Source: CAD feature listing. Evaluate the final solid. Frame: model axes, mm. A direction names the side the tool comes from. Coordinates: 2 decimals unless noted, no trailing zeros. Order: outer loops, then holes, each group sorted by start corner. A loop starts at its lowest first (then second) coordinate and runs counter-clockwise, first axis right, second up. Notation, with made-up numbers: (41.25, 26.25) -> (97.25, 26.25) arc R22 ccw to (97.25, 57.25) -> close; hole circle Ø2 at (53, 75). An arc over 180 degrees is marked (long way). Put each result on its own line as item: value.
from build123d import *

# Parameters (mm, degrees)
SKETCH_W        = 50
SKETCH_H        = 55
PAD_DEPTH       = 4
PAD001_DEPTH    = 50
SKETCH002_R     = 11
POCKET_DEPTH    = 5
SKETCH003_R     = 1.6
POCKET001_DEPTH = 50
SKETCH004_W     = 54
SKETCH004_H     = 63
PAD002_DEPTH    = 4
SKETCH005_R     = 2.1
POCKET002_DEPTH = 60
POCKET003_DEPTH = 5
POCKET004_DEPTH = 70
SKETCH008_W     = 45
SKETCH008_H     = 45
POCKET005_DEPTH = 5


with BuildPart() as part:
    # Sketch → Pad (new body)
    with BuildSketch(Plane.XY):
        with Locations((25, 27.5)):
            Rectangle(SKETCH_W, SKETCH_H)
    extrude(amount=PAD_DEPTH)

    # Sketch001 (on Face6 of Pad) → Pad001 (join)
    with BuildSketch(Plane.XY.offset(4)):
        Polygon((50, 55), (50, 59), (-4, 59), (-4, -4), (50, -4), (50, 0), (0, 0), (0, 55), align=None)
    extrude(amount=-PAD001_DEPTH)

    # Sketch002 (on Face4 of Pad001) → Pocket (cut)
    with BuildSketch(Plane(origin=(0, 0, 0), x_dir=(1, 0, 0), z_dir=(0, 0, -1))):
        with Locations((25, -25)):
            Circle(SKETCH002_R)
    extrude(amount=-POCKET_DEPTH, mode=Mode.SUBTRACT)

    # Sketch003 (on Face5 of Pocket) → Pocket001 (cut)
    with BuildSketch(Plane.XY.offset(4)):
        with Locations((40.5, 40.5)):
            Circle(SKETCH003_R)
        with Locations((40.5, 9.5)):
            Circle(SKETCH003_R)
        with Locations((9.5, 9.5)):
            Circle(SKETCH003_R)
        with Locations((9.5, 40.5)):
            Circle(SKETCH003_R)
    extrude(amount=-POCKET001_DEPTH, mode=Mode.SUBTRACT)

    # Sketch004 (on DatumPlane) → Pad002 (join)
    with BuildSketch(Plane(origin=(0, 0, -46), x_dir=(1, 0, 0), z_dir=(0, 0, -1))):
        with Locations((23, -27.5)):
            Rectangle(SKETCH004_W, SKETCH004_H)
    extrude(amount=PAD002_DEPTH)

    # Sketch005 (on Face22 of Pad002) → Pocket002 (cut)
    with BuildSketch(Plane(origin=(0, 0, -50), x_dir=(1, 0, 0), z_dir=(0, 0, -1))):
        with Locations((5, -5)):
            Circle(SKETCH005_R)
        with Locations((45, -5)):
            Circle(SKETCH005_R)
        with Locations((45, -51)):
            Circle(SKETCH005_R)
        with Locations((5, -51)):
            Circle(SKETCH005_R)
    extrude(amount=-POCKET002_DEPTH, mode=Mode.SUBTRACT)

    # Sketch006 (on Face22 of Pocket002) → Pocket003 (cut)
    with BuildSketch(Plane(origin=(-4, 0, 0), x_dir=(0, -1, 0), z_dir=(-1, 0, 0))):
        with BuildLine():
            ThreePointArc((-48, -10), (-49.5, -11.5), (-48, -13))
            Line((-48, -13), (-8, -13))
            ThreePointArc((-8, -13), (-6.5, -11.5), (-8, -10))
            Line((-8, -10), (-48, -10))
        make_face()
        with BuildLine():
            ThreePointArc((-48, -24.994244), (-49.5, -26.494244), (-48, -27.994244))
            Line((-48, -27.994244), (-8, -27.994244))
            ThreePointArc((-8, -27.994244), (-6.5, -26.494244), (-8, -24.994244))
            Line((-8, -24.994244), (-48, -24.994244))
        make_face()
        with BuildLine():
            ThreePointArc((-47.876909, -14.998485), (-49.376909, -16.498485), (-47.876909, -17.998485))
            Line((-47.876909, -17.998485), (-7.876909, -17.998485))
            ThreePointArc((-7.876909, -17.998485), (-6.376909, -16.498485), (-7.876909, -14.998485))
            Line((-7.876909, -14.998485), (-47.876909, -14.998485))
        make_face()
        with BuildLine():
            ThreePointArc((-48.0704, -19.994739), (-49.5704, -21.494739), (-48.0704, -22.994739))
            Line((-48.0704, -22.994739), (-8.0704, -22.994739))
            ThreePointArc((-8.0704, -22.994739), (-6.5704, -21.494739), (-8.0704, -19.994739))
            Line((-8.0704, -19.994739), (-48.0704, -19.994739))
        make_face()
        with BuildLine():
            ThreePointArc((-48, -34.994244), (-49.5, -36.494244), (-48, -37.994244))
            Line((-48, -37.994244), (-8, -37.994244))
            ThreePointArc((-8, -37.994244), (-6.5, -36.494244), (-8, -34.994244))
            Line((-8, -34.994244), (-48, -34.994244))
        make_face()
        with BuildLine():
            ThreePointArc((-48, -29.994244), (-49.5, -31.494244), (-48, -32.994244))
            Line((-48, -32.994244), (-8, -32.994244))
            ThreePointArc((-8, -32.994244), (-6.5, -31.494244), (-8, -29.994244))
            Line((-8, -29.994244), (-48, -29.994244))
        make_face()
    extrude(amount=-POCKET003_DEPTH, mode=Mode.SUBTRACT)

    # Sketch007 (on Face11 of Pocket003) → Pocket004 (cut)
    with BuildSketch(Plane(origin=(0, 59, 0), x_dir=(-1, 0, 0), z_dir=(0, 1, 0))):
        with BuildLine():
            ThreePointArc((-35, -8.5), (-36.5, -10), (-35, -11.5))
            Line((-35, -11.5), (-10, -11.5))
            ThreePointArc((-10, -11.5), (-8.5, -10), (-10, -8.5))
            Line((-10, -8.5), (-35, -8.5))
        make_face()
        with BuildLine():
            ThreePointArc((-35, -14.5), (-36.5, -16), (-35, -17.5))
            Line((-35, -17.5), (-10, -17.5))
            ThreePointArc((-10, -17.5), (-8.5, -16), (-10, -14.5))
            Line((-10, -14.5), (-35, -14.5))
        make_face()
        with BuildLine():
            ThreePointArc((-35, -20.53228), (-36.5, -22.03228), (-35, -23.53228))
            Line((-35, -23.53228), (-10, -23.53228))
            ThreePointArc((-10, -23.53228), (-8.5, -22.03228), (-10, -20.53228))
            Line((-10, -20.53228), (-35, -20.53228))
        make_face()
        with BuildLine():
            ThreePointArc((-35, -26.484331), (-36.5, -27.984331), (-35, -29.484331))
            Line((-35, -29.484331), (-10, -29.484331))
            ThreePointArc((-10, -29.484331), (-8.5, -27.984331), (-10, -26.484331))
            Line((-10, -26.484331), (-35, -26.484331))
        make_face()
        with BuildLine():
            ThreePointArc((-35, -32.449028), (-36.5, -33.949028), (-35, -35.449028))
            Line((-35, -35.449028), (-10, -35.449028))
            ThreePointArc((-10, -35.449028), (-8.5, -33.949028), (-10, -32.449028))
            Line((-10, -32.449028), (-35, -32.449028))
        make_face()
        with BuildLine():
            ThreePointArc((-35, -38.428181), (-36.5, -39.928181), (-35, -41.428181))
            Line((-35, -41.428181), (-10, -41.428181))
            ThreePointArc((-10, -41.428181), (-8.5, -39.928181), (-10, -38.428181))
            Line((-10, -38.428181), (-35, -38.428181))
        make_face()
    extrude(amount=-POCKET004_DEPTH, mode=Mode.SUBTRACT)

    # Sketch008 (on Face50 of Pocket004) → Pocket005 (cut)
    with BuildSketch(Plane(origin=(0, 0, -50), x_dir=(1, 0, 0), z_dir=(0, 0, -1))):
        with Locations((25, -25)):
            Rectangle(SKETCH008_W, SKETCH008_H)
    extrude(amount=-POCKET005_DEPTH, mode=Mode.SUBTRACT)


solid = part.part
1. First-contact query: pin 1 (3 mm diameter, centred on y = 52.5, z = -13, fed in from +X); pin 2 (15 mm diameter, centred on x = 31, y = 30.5, fed in from -Z). Flat tips, straight axial feed; report the tip coordinate or a pass-through.
Numbers:
pin 1: stops at x = 0
pin 2: stops at z = 0
2. Cut plane A-A on x = 40.5. Output: boundary loops of the cut face in (y, z).
Numbers:
outline: (-4, -50) -> (2.5, -50) -> (2.5, -46) -> (0, -46) -> (0, 0) -> (7.9, 0) -> (7.9, 4) -> (-4, 4) -> close; (11.1, 0) -> (38.9, 0) -> (38.9, 4) -> (11.1, 4) -> close; (42.1, 0) -> (55, 0) -> (55, -46) -> (47.5, -46) -> (47.5, -50) -> (59, -50) -> (59, 4) -> (42.1, 4) -> close
3. Set-up query: faces 4 (the flat face through (-2, 28, -10)), 5 (the cylindrical face through (8.5, -2, -40)), 6 (the cylindrical face through (45.969, 52.863, -48.028)). Return all of +Z, -Z, +X, -X, +Y, -Y with unobstructed straight access to the full face (end or side cutting, diameter ignored); none if empty.
Numbers:
face 4: +X, -X
face 5: +Y, -Y
face 6: +Z, -Z
4. Cut plane B-B on z = -40. Output: boundary loops of the cut face in (x, y).
Numbers:
outline: (-4, -4) -> (8.5, -4) -> (8.5, 0) -> (0, 0) -> (0, 55) -> (8.5, 55) -> (8.5, 59) -> (-4, 59) -> close; (36.5, -4) -> (50, -4) -> (50, 0) -> (36.5, 0) -> close; (36.5, 55) -> (50, 55) -> (50, 59) -> (36.5, 59) -> close
5. Cut plane D-D on x = 25. Count the separate pieces of the cut face and the enclosed holes in it, plus the area to 3 significant figures.
Numbers:
separate pieces: 14
enclosed holes: 0
area: 460 mm2
6. Ray query, line 1 along Y through (x, z) = (45, -48.65); line 2 along Y through (x, z) = (40.5, 2.05); line 3 along X through (y, z) = (5, 2). Return the intervals inside material, ascending.
Numbers:
line 1: y = -4 to 2.5, 47.5 to 48.9, 53.1 to 59
line 2: y = -4 to 7.9, 11.1 to 38.9, 42.1 to 59
line 3: x = -4 to 2.9, 7.1 to 42.9, 47.1 to 50
7. Pull-direction query (Y, two-part tool) for faces 1 (the flat face through (22, 57, -32.449)), 2 (the cylindrical face through (-2.03, 49.57, -21.46)), 3 (the flat face through (23, -4, -5)); classes: pulls with the +Y half, pulls with the -Y half, needs draft (parallel to the pull), parting line crosses it, or undercut.
Numbers:
face 1: needs draft
face 2: undercut
face 3: pulls with the -Y half
8. Cut plane C-C on z = -16. Output: boundary loops of the cut face in (x, y), plus the area to 3 significant figures.
Numbers:
outline: (-4, -4) -> (8.5, -4) -> (8.5, 0) -> (0, 0) -> (0, 6.46) -> (-4, 6.46) -> close; (-4, 49.29) -> (0, 49.29) -> (0, 55) -> (8.5, 55) -> (8.5, 59) -> (-4, 59) -> close; (36.5, -4) -> (50, -4) -> (50, 0) -> (36.5, 0) -> close; (36.5, 55) -> (50, 55) -> (50, 59) -> (36.5, 59) -> close
area: 257 mm2
